Could you check a few things on this model? Use its own coordinates, in mm. Coordinates: 2 decimals unless noted, no trailing zeros. Order: outer loops, then holes, each group sorted by start corner. A loop starts at its lowest first (then second) coordinate and runs counter-clockwise, first axis right, second up. Notation, with made-up numbers: (-32.75, -8.5) - (-3.75, -8.5) arc R19 cw to (-3.75, -1.5) - close; hole circle Ø11 at (-7, 85.5). An arc over 180 degrees is marked (long way). One line per item, written item: value.
from build123d import *

# Parameters (mm, degrees)
F0_R     = 11.35
F1_DEPTH = 7


# Not quite as in the source:
# - a feature names something its author has since deleted; it is built from what else it names


with BuildPart() as f1:
    # F0 (on Top) → F1 (new body)
    with BuildSketch(Plane.XY):
        with BuildLine():
            ThreePointArc((0, -15), (10.6066017178, -10.6066017178), (15, 0))
            ThreePointArc((15, 0), (10.6066016959, 10.6066017397), (-6.18e-08, 15))
            ThreePointArc((-6.18e-08, 15), (-10.6066017397, 10.6066016959), (-15, 0))
            ThreePointArc((-15, 0), (-10.6066017178, -10.6066017178), (0, -15))
        make_face()
        Circle(F0_R, mode=Mode.SUBTRACT)
        with BuildLine():
            ThreePointArc((15, -30), (19.0192378865, -15), (15, 0))
            ThreePointArc((15, 0), (10.6066017178, -10.6066017178), (0, -15))
            ThreePointArc((0, -15), (10.6066017178, -19.3933982822), (15, -30))
        make_face()
        with BuildLine():
            ThreePointArc((-6.18e-08, 15), (10.6066016959, 10.6066017397), (15, 0))
            ThreePointArc((15, 0), (19.0192378865, 15), (15, 30))
            ThreePointArc((15, 30), (10.6066016959, 19.3933982603), (-6.18e-08, 15))
        make_face()
        with BuildLine():
            ThreePointArc((-15, 0), (-10.6066017397, 10.6066016959), (-6.18e-08, 15))
            ThreePointArc((-6.18e-08, 15), (-10.6066017397, 19.3933983041), (-15, 30))
            ThreePointArc((-15, 30), (-19.0192378865, 15), (-15, 0))
        make_face()
        with BuildLine():
            ThreePointArc((-15, 30), (-10.6066017397, 19.3933983041), (-6.18e-08, 15))
            ThreePointArc((-6.18e-08, 15), (10.6066016959, 19.3933982603), (15, 30))
            ThreePointArc((15, 30), (0, 45), (-15, 30))
        make_face()
        with Locations((0, 30)):
            Circle(F0_R, mode=Mode.SUBTRACT)
        with BuildLine():
            ThreePointArc((-15, -30), (-10.6066017178, -19.3933982822), (0, -15))
            ThreePointArc((0, -15), (-10.6066017178, -10.6066017178), (-15, 0))
            ThreePointArc((-15, 0), (-19.0192378865, -15), (-15, -30))
        make_face()
        with BuildLine():
            ThreePointArc((15, -30), (10.6066017178, -19.3933982822), (0, -15))
            ThreePointArc((0, -15), (-10.6066017178, -19.3933982822), (-15, -30))
            ThreePointArc((-15, -30), (0, -45), (15, -30))
        make_face()
        with Locations((0, -30)):
            Circle(F0_R, mode=Mode.SUBTRACT)
    extrude(amount=F1_DEPTH)


solid = f1.part
Item 1: If I drill on probe 1 along Y at (x, z) = (0, 2); probe 2 along Y at (x, z) = (3, 2); probe 3 along X at (y, z) = (23.5, 2.5), over which ranges is the centre line in solid material (lowest first)?
Conclusion:
probe 1: -45 to -41.35, -18.65 to -11.35, 11.35 to 18.65, 41.35 to 45
probe 2: -44.7 to -40.95, -19.05 to -10.95, 10.95 to 19.05, 40.95 to 44.7
probe 3: -17.79 to -9.3, 9.3 to 17.79
Item 2: I want a section at D-D on x = 4.5. Please give me the cut outline in (y, z).
Conclusion:
outline: (-44.31, 0) - (-40.42, 0) - (-40.42, 7) - (-44.31, 7) - close; (-19.58, 0) - (-10.42, 0) - (-10.42, 7) - (-19.58, 7) - close; (10.42, 0) - (19.58, 0) - (19.58, 7) - (10.42, 7) - close; (40.42, 0) - (44.31, 0) - (44.31, 7) - (40.42, 7) - close
Item 3: I want a section at C-C on y = -23. Please give me the cut outline in (x, z).
Conclusion:
outline: (-17.93, 0) - (-8.93, 0) - (-8.93, 7) - (-17.93, 7) - close; (8.93, 0) - (17.93, 0) - (17.93, 7) - (8.93, 7) - close
Item 4: Thinking about a two-plate mould opening in X: for faces 1 (the face through (10.485, 25.653, 3.451)), 2 (the face through (0, -45, 3)), 3 (the face through (-19.02, 15.22, 3.45)), 4 (the face through (-4, 11, 0)), which applies, pulls with the +X half, pulls with the -X half, needs draft (parallel to the pull), parting line crosses it, or undercut?
Conclusion:
face 1: undercut
face 2: parting line crosses it
face 3: pulls with the -X half
face 4: needs draft
Item 5: I'm going to push flat-ended pins straight in: pin 1 Ø4 at (x, z) = (-11, 5) entering from +Y; pin 2 Ø1.5 at (y, z) = (33, 6) entering from +X; pin 3 Ø3 at (y, z) = (36, 1.5) entering from -X; pin 4 Ø4 at (x, y) = (7.5, -5.5) entering from +Z. Where does each tip first touch, or does it pass through?
Conclusion:
pin 1: y = 42
pin 2: x = 14.83
pin 3: x = -14.31
pin 4: through
Item 6: I want a section at A-A on z = 1. Please give me the cut outline in (x, y).
Conclusion:
outline: (-15, -30) arc R15 ccw to (15, -30) arc R30 ccw to (15, 0) arc R30 ccw to (15, 30) arc R15 ccw to (-15, 30) arc R30 ccw to (-15, 0) arc R30 ccw to start; hole circle Ø22.7 at (0, -30); hole circle Ø22.7 at (0, 0); hole circle Ø22.7 at (0, 30)
Item 7: I want a section at B-B on x = 0. Please give me the cut outline in (y, z), then the cut area to 3 significant figures.
Conclusion:
outline: (-45, 0) - (-41.35, 0) - (-41.35, 7) - (-45, 7) - close; (-18.65, 0) - (-11.35, 0) - (-11.35, 7) - (-18.65, 7) - close; (11.35, 0) - (18.65, 0) - (18.65, 7) - (11.35, 7) - close; (41.35, 0) - (45, 0) - (45, 7) - (41.35, 7) - close
area: 153 mm²
